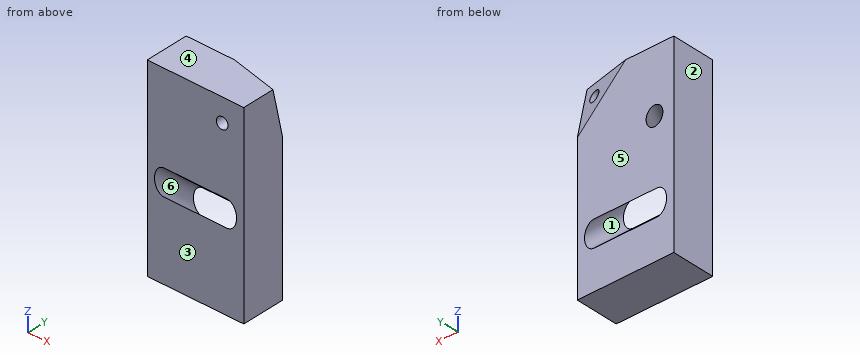
from build123d import *

# Parameters (mm, degrees)
SKETCH1_W           = 200
SKETCH1_H           = 400
BOSS_EXTRUDE1_DEPTH = 90
CUT_EXTRUDE2_DEPTH  = 289.26854046
SKETCH4_3_R         = 11.813497964
CUT_EXTRUDE4_DEPTH  = 289.26854046
SKETCH10_RX         = 20
SKETCH10_RY         = 15
CUT_EXTRUDE5_DEPTH  = 100
CUT_EXTRUDE6_DEPTH  = 380.479144091


with BuildPart() as part:
    # Sketch1 → Boss-Extrude1 (new body)
    with BuildSketch(Plane(origin=(0, 0, 0), x_dir=(1, 0, 0), z_dir=(0, 1, 0))):
        Rectangle(SKETCH1_W, SKETCH1_H)
    extrude(amount=BOSS_EXTRUDE1_DEPTH)

    # Sketch4 → Cut-Extrude2 (cut, through all)
    with BuildSketch(Plane(origin=(27.582292849, 122.587968218, 27.582292849), x_dir=(-0.9767443431718839, 0.20917784862693525, 0.04706501594106042), z_dir=(-0.21440729484260865, -0.9529213104115941, -0.21440729484260865))):
        Polygon((28.239009565, -175.365853659), (-74.141926347, -77.804878049), (-74.141926347, -180.304878049), align=None)
    extrude(amount=-CUT_EXTRUDE2_DEPTH, mode=Mode.SUBTRACT)

    # Sketch4_3 → Cut-Extrude4 (cut, through all)
    with BuildSketch(Plane(origin=(27.582292849, 122.587968218, 27.582292849), x_dir=(-0.9767443431718839, 0.20917784862693525, 0.04706501594106042), z_dir=(-0.21440729484260865, -0.9529213104115941, -0.21440729484260865))):
        with Locations(Location((-46.760990435, -147.804878049, 0), (0, 0, 226.380950612))):
            Circle(SKETCH4_3_R)
    extrude(amount=CUT_EXTRUDE4_DEPTH, mode=Mode.SUBTRACT)

    # Sketch10 → Cut-Extrude5 (cut)
    with BuildSketch(Plane(origin=(-63.97114317, 110.801270189, 0), x_dir=(0, 0, 1), z_dir=(-0.500000000000001, 0.866025403784438, 0))):
        with Locations(Location((70, -6.961524227), (0, 0, 180))):
            Ellipse(SKETCH10_RX, SKETCH10_RY)
    extrude(amount=-CUT_EXTRUDE5_DEPTH, mode=Mode.SUBTRACT)

    # Sketch11 → Cut-Extrude6 (cut, through all)
    with BuildSketch(Plane(origin=(0, 149.155970384, -134.300638965), x_dir=(-1, 0, 0), z_dir=(0, 0.7431448254773932, -0.6691306063588595))):
        with BuildLine():
            Line((-65, 11.592789477), (65, 11.592789477))
            ThreePointArc((65, 11.592789477), (85, -8.407210523), (65, -28.407210523))
            Line((65, -28.407210523), (-65, -28.407210523))
            ThreePointArc((-65, -28.407210523), (-85, -8.407210523), (-65, 11.592789477))
        make_face()
    extrude(amount=-CUT_EXTRUDE6_DEPTH, mode=Mode.SUBTRACT)


solid = part.part
Read the model definition and answer for the solid it produces. Units are mm, in the model's axes. Face numbers are marked on the shaded views. A direction names the side the tool comes from. Coordinates: 2 decimals unless noted, no trailing zeros. Put each result on its own line as item: value. Start each with the question number.
Item 1: Consider probe 1 along Z at (x, y) = (69, 74); probe 2 along Z at (x, y) = (65, 57.5); probe 3 along Y at (x, z) = (39.5, -42.5). Determine where each line is inside the solid, lowest interval first. Write a range as [from, to].
Item 2: The mould has two halves that part along Y. Classify the marked faces 3, 4, 5 and 6: +Y half, -Y half, draft (parallel to the pull), parting line (faces both ways), or undercut.
Item 3: Section A-A, the plane x = -14.5 is taken. Count the separate pieces of the cut face and the enclosed holes in it, plus the area to 3 significant figures.
Item 4: For the marked faces 1 and 2, determine the directions among +Z, -Z, +X, -X, +Y, -Y from which every point of the face is accessible in a straight line to the end or side of a thin tool.
Computed:
1. probe 1: z = [-200, -104.31], [-51.57, 156.25], [179.78, 200]
1. probe 2: z = [-200, -90], [-36.17, 152.6], [175.98, 200]
1. probe 3: y = [0, 4.75], [64.53, 90]
2. face 3: -Y half
2. face 4: draft
2. face 5: +Y half
2. face 6: undercut
3. separate pieces: 2
3. enclosed holes: 1
3. area: 30,700 mm2
4. face 1: none
4. face 2: +Z, -Z, -X, +Y, -Y
